```python
from build123d import *

# Parameters (mm, degrees)
SKETCH1_R           = 30.25
SKETCH1_R_2         = 25.25
EXTRUDE_THIN1_DEPTH = 3
SKETCH2_R           = 1.65
CUT_EXTRUDE3_DEPTH  = 10
BOSS_EXTRUDE1_DEPTH = 3


with BuildPart() as part:
    # Sketch1 → Extrude-Thin1 (new body)
    with BuildSketch(Plane(origin=(0, 0, 0), x_dir=(1, 0, 0), z_dir=(0, 1, 0))):
        Circle(SKETCH1_R)
        Circle(SKETCH1_R_2, mode=Mode.SUBTRACT)
    extrude(amount=-EXTRUDE_THIN1_DEPTH)

    # Sketch2 → Cut-Extrude3 (cut)
    with BuildSketch(Plane(origin=(0, 0, 0), x_dir=(1, 0, 0), z_dir=(0, 1, 0))):
        with Locations((0, 27.5)):
            Circle(SKETCH2_R)
        with Locations((23.815698604, -13.75)):
            Circle(SKETCH2_R)
        with Locations((-23.815698604, -13.75)):
            Circle(SKETCH2_R)
    extrude(amount=-CUT_EXTRUDE3_DEPTH, mode=Mode.SUBTRACT)

    # Sketch5 → Boss-Extrude1 (add)
    with BuildSketch(Plane.XZ.offset(3)):
        with BuildLine():
            Line((0, 42.25), (0, 30.25))
            ThreePointArc((0, 30.25), (2.636461218, 30.134889617), (5.252857374, 29.790434529))
            Line((5.252857374, 29.790434529), (7.336635506, 41.608127565))
            ThreePointArc((7.336635506, 41.608127565), (3.682330131, 42.089225994), (0, 42.25))
        make_face()
        with BuildLine():
            Line((19.634554019, 37.410517084), (14.057875954, 26.785044776))
            ThreePointArc((14.057875954, 26.785044776), (16.338851964, 25.457894974), (18.495479445, 23.936995219))
            Line((18.495479445, 23.936995219), (25.832529142, 33.432662744))
            ThreePointArc((25.832529142, 33.432662744), (22.820380016, 35.556894633), (19.634554019, 37.410517084))
        make_face()
        with BuildLine():
            Line((34.771068334, 24.000735549), (24.895261943, 17.183958589))
            ThreePointArc((24.895261943, 17.183958589), (26.29820863, 14.948803393), (27.501010069, 12.599878777))
            Line((27.501010069, 12.599878777), (38.410501667, 17.598177795))
            ThreePointArc((38.410501667, 17.598177795), (36.730555855, 20.878907218), (34.771068334, 24.000735549))
        make_face()
        with BuildLine():
            Line((41.941949931, 5.092674741), (30.029443441, 3.646234578))
            ThreePointArc((30.029443441, 3.646234578), (30.232962626, 1.015121107), (30.20639071, -1.623718049))
            Line((30.20639071, -1.623718049), (42.189091156, -2.267837605))
            ThreePointArc((42.189091156, -2.267837605), (42.226203998, 1.417813777), (41.941949931, 5.092674741))
        make_face()
        with BuildLine():
            Line((39.504436253, -14.982056478), (28.284241341, -10.726797833))
            ThreePointArc((28.284241341, -10.726797833), (27.241709231, -13.151113191), (25.991851265, -15.475340637))
            Line((25.991851265, -15.475340637), (36.302668296, -21.61431874))
            ThreePointArc((36.302668296, -21.61431874), (38.048337687, -18.368083713), (39.504436253, -14.982056478))
        make_face()
        with BuildLine():
            Line((28.016932311, -31.62457911), (20.059460412, -22.642450132))
            ThreePointArc((20.059460412, -22.642450132), (18.00970855, -24.304585945), (15.822891931, -25.781749183))
            Line((15.822891931, -25.781749183), (22.099741623, -36.009219933))
            ThreePointArc((22.099741623, -36.009219933), (25.154055743, -33.946074584), (28.016932311, -31.62457911))
        make_face()
        with BuildLine():
            Line((10.111086816, -41.022291786), (7.239298845, -29.370989977))
            ThreePointArc((7.239298845, -29.370989977), (4.65190068, -29.890170961), (2.029098743, -30.181869695))
            Line((2.029098743, -30.181869695), (2.834030476, -42.154842797))
            ThreePointArc((2.834030476, -42.154842797), (6.497282768, -41.747428862), (10.111086816, -41.022291786))
        make_face()
        with BuildLine():
            Line((-10.111086816, -41.022291786), (-7.239298845, -29.370989977))
            ThreePointArc((-7.239298845, -29.370989977), (-9.771601574, -28.628278025), (-12.229536514, -27.667687591))
            Line((-12.229536514, -27.667687591), (-17.0809229, -38.643299198))
            ThreePointArc((-17.0809229, -38.643299198), (-13.647939388, -39.9849503), (-10.111086816, -41.022291786))
        make_face()
        with BuildLine():
            Line((-28.016932311, -31.62457911), (-20.059460412, -22.642450132))
            ThreePointArc((-20.059460412, -22.642450132), (-21.956547668, -20.807991602), (-23.686532338, -18.815171692))
            Line((-23.686532338, -18.815171692), (-33.082842687, -26.279041454))
            ThreePointArc((-33.082842687, -26.279041454), (-30.666583106, -29.062401494), (-28.016932311, -31.62457911))
        make_face()
        with BuildLine():
            Line((-39.504436253, -14.982056478), (-28.284241341, -10.726797833))
            ThreePointArc((-28.284241341, -10.726797833), (-29.111513296, -8.220845067), (-29.717229057, -5.652326705))
            Line((-29.717229057, -5.652326705), (-41.505881906, -7.89457201))
            ThreePointArc((-41.505881906, -7.89457201), (-40.659882207, -11.482006746), (-39.504436253, -14.982056478))
        make_face()
        with BuildLine():
            Line((-41.941949931, 5.092674741), (-30.029443441, 3.646234578))
            ThreePointArc((-30.029443441, 3.646234578), (-29.59738206, 6.249598002), (-28.94006673, 8.805398211))
            Line((-28.94006673, 8.805398211), (-40.42042378, 12.298448742))
            ThreePointArc((-40.42042378, 12.298448742), (-41.338492299, 8.728777374), (-41.941949931, 5.092674741))
        make_face()
        with BuildLine():
            Line((-34.771068334, 24.000735549), (-24.895261943, 17.183958589))
            ThreePointArc((-24.895261943, 17.183958589), (-23.302847281, 19.288333484), (-21.533083881, 21.245912515))
            Line((-21.533083881, 21.245912515), (-30.075133685, 29.674043099))
            ThreePointArc((-30.075133685, 29.674043099), (-32.546951988, 26.939903791), (-34.771068334, 24.000735549))
        make_face()
        with BuildLine():
            Line((-19.634554019, 37.410517084), (-14.057875954, 26.785044776))
            ThreePointArc((-14.057875954, 26.785044776), (-11.66991102, 27.908344214), (-9.193131017, 28.819244302))
            Line((-9.193131017, 28.819244302), (-12.839992908, 40.251671793))
            ThreePointArc((-12.839992908, 40.251671793), (-16.29929721, 38.979422911), (-19.634554019, 37.410517084))
        make_face()
    extrude(amount=-BOSS_EXTRUDE1_DEPTH)


solid = part.part
```
Part model, mm, in its own coordinate system. A direction names the side the tool comes from. Coordinates: 2 decimals unless noted, no trailing zeros. Write each loop counter-clockwise with the first axis right and the second up, starting at its lowest first coordinate (ties: lowest second). Pieces come first, ordered by that corner, then holes.
Item 1: Slice it at A-A (z = 0). Write the cut outline in (x, y), and give its area (3 significant figures).
Item 2: Mould opens along X. For faces 1 (the face through (-24.094, -1.521, -27.196)), 2 (the face through (-14.62, -1.52, -33.08)), 3 (the face through (36.76, -1.52, 20.83)), 4 (the face through (-32.514, -1.521, 26.98)) say: released by +X, released by -X, zero draft, split by the parting line, or undercut.
Item 3: Which spindle directions (+Z, -Z, +X, -X, +Y, -Y) get a long thin tool onto all of the face, cutting with end or side? Do faces 5 (the face through (-41.328, -1.521, 8.779)), 6 (the face through (-18.062, -1.479, 24.266)), 7 (the face through (-4.72, -1.48, 29.88)). Say none if no direction does.
Item 4: Slice it at B-B (z = -12.5). Write the cut outline in (x, y).
Item 5: Pin check, flat tip, straight feed: pin 1 (1.5 mm diameter, centred on y = -2, z = 34, fed in from -X). Stop position of the tip, or through.
Item 6: Slice it at D-D (z = 13.75). Write the cut outline in (x, y).
Item 7: Probe line 1 (X direction, y = -1.65, z = -1); line 2 (Z direction, x = -1.5, y = -1.25); line 3 (X direction, y = -1.1, z = -27.5). List the from-to ranges inside material, lowest first.
Item 8: Slice it at C-C (x = 12). Write the cut outline in (y, z), and give its area (3 significant figures).
Results found:
1. outline: (-30.25, -3) - (-25.25, -3) - (-25.25, 0) - (-30.25, 0) - close; (25.25, -3) - (42.25, -3) - (42.25, 0) - (25.25, 0) - close
1. area: 66.0 mm2
2. face 1: undercut
2. face 2: undercut
2. face 3: released by +X
2. face 4: released by -X
3. face 5: +Z, -X, +Y, -Y
3. face 6: +Y, -Y
3. face 7: +Z, +Y, -Y
4. outline: (-40.36, -3) - (-32.96, -3) - (-32.96, 0) - (-40.36, 0) - close; (-27.55, -3) - (-21.94, -3) - (-21.94, 0) - (-27.55, 0) - close; (21.94, -3) - (32.96, -3) - (32.96, 0) - (21.94, 0) - close
5. pin 1: stops at x = -18.24
6. outline: (-26.94, -3) - (-25.47, -3) - (-25.47, 0) - (-26.94, 0) - close; (-22.17, -3) - (-21.18, -3) - (-21.18, 0) - (-22.17, 0) - close; (21.18, -3) - (22.17, -3) - (22.17, 0) - (21.18, 0) - close; (25.47, -3) - (30.01, -3) - (30.01, 0) - (25.47, 0) - close
7. line 1: x = -30.23 to -25.23, 25.23 to 42.24
7. line 2: z = -30.21 to -28.19, -26.81 to -25.21, 25.21 to 30.21
7. line 3: x = -32.08 to -24.36, -12.6 to -1.65, 1.65 to 12.6, 16.88 to 24.36
8. outline: (-3, -27.77) - (0, -27.77) - (0, -22.22) - (-3, -22.22) - close; (-3, 22.22) - (0, 22.22) - (0, 27.77) - (-3, 27.77) - close
8. area: 33.3 mm2
